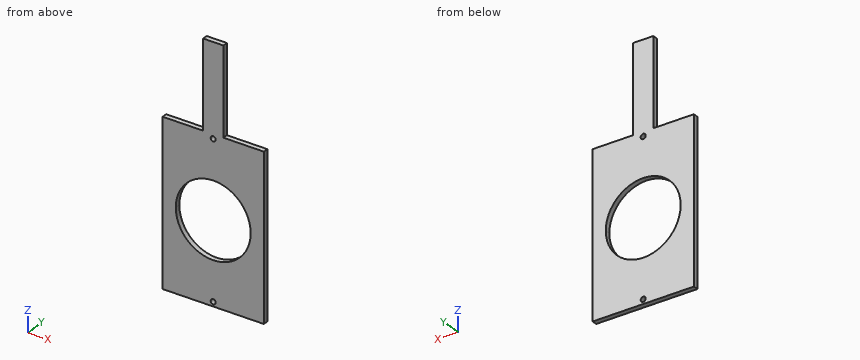
from build123d import *

# Parameters (mm, degrees)
F1_DEPTH = 3.175


# Not quite as in the source:
# - a feature names something its author has since deleted; it is built from what else it names


with BuildPart() as f1:
    # F0 (on Front) → F1 (new body)
    with BuildSketch(Plane.XZ):
        with BuildLine():
            Line((-94.8762850642, 108.0007998444), (-120.2762850642, 108.0007998444))
            Line((-120.2762850642, 108.0007998444), (-120.2762850642, 57.2007998444))
            Line((-120.2762850642, 57.2007998444), (-112.0251095462, 57.2007998444))
            ThreePointArc((-112.0251095462, 57.2007998444), (-105.1424632053, 73.8169779855), (-88.5262850642, 80.6996243264))
            Line((-88.5262850642, 80.6996243264), (-88.5262850642, 103.6132998444))
            ThreePointArc((-88.5262850642, 103.6132998444), (-90.1137850642, 105.2007998444), (-88.5262850642, 106.7882998444))
            Line((-88.5262850642, 106.7882998444), (-88.5262850642, 108.0007998444))
            Line((-88.5262850642, 108.0007998444), (-94.8762850642, 108.0007998444))
        make_face()
        with BuildLine():
            Line((-82.1762850642, 108.0007998444), (-88.5262850642, 108.0007998444))
            Line((-88.5262850642, 108.0007998444), (-88.5262850642, 106.7882998444))
            ThreePointArc((-88.5262850642, 106.7882998444), (-87.4037530491, 106.3233318595), (-86.9387850642, 105.2007998444))
            ThreePointArc((-86.9387850642, 105.2007998444), (-87.4037530491, 104.0782678293), (-88.5262850642, 103.6132998444))
            Line((-88.5262850642, 103.6132998444), (-88.5262850642, 80.6996243264))
            ThreePointArc((-88.5262850642, 80.6996243264), (-71.9101069231, 73.8169779855), (-65.0274605822, 57.2007998444))
            ThreePointArc((-65.0274605822, 57.2007998444), (-71.9101069231, 40.5846217033), (-88.5262850642, 33.7019753624))
            Line((-88.5262850642, 33.7019753624), (-88.5262850642, 10.7882998444))
            ThreePointArc((-88.5262850642, 10.7882998444), (-87.4037530491, 10.3233318595), (-86.9387850642, 9.2007998444))
            ThreePointArc((-86.9387850642, 9.2007998444), (-87.4037530491, 8.0782678293), (-88.5262850642, 7.6132998444))
            Line((-88.5262850642, 7.6132998444), (-88.5262850642, 6.4007998444))
            Line((-88.5262850642, 6.4007998444), (-56.7762850642, 6.4007998444))
            Line((-56.7762850642, 6.4007998444), (-56.7762850642, 108.0007998444))
            Line((-56.7762850642, 108.0007998444), (-82.1762850642, 108.0007998444))
        make_face()
        with BuildLine():
            Line((-112.0251095462, 57.2007998444), (-120.2762850642, 57.2007998444))
            Line((-120.2762850642, 57.2007998444), (-120.2762850642, 6.4007998444))
            Line((-120.2762850642, 6.4007998444), (-88.5262850642, 6.4007998444))
            Line((-88.5262850642, 6.4007998444), (-88.5262850642, 7.6132998444))
            ThreePointArc((-88.5262850642, 7.6132998444), (-90.1137850642, 9.2007998444), (-88.5262850642, 10.7882998444))
            Line((-88.5262850642, 10.7882998444), (-88.5262850642, 33.7019753624))
            ThreePointArc((-88.5262850642, 33.7019753624), (-105.1424632053, 40.5846217033), (-112.0251095462, 57.2007998444))
        make_face()
        Polygon((-94.8762850642, 162.3507998444), (-94.8762850642, 108.0007998444), (-88.5262850642, 108.0007998444), (-82.1762850642, 108.0007998444), (-82.1762850642, 162.3507998444), align=None)
    extrude(amount=F1_DEPTH)


solid = f1.part
The listing builds one solid part. Answer for the finished solid, in the listing's coordinates (mm). Give positions to 0.01 mm unless a question says otherwise; leave off trailing zeros. Order: outer loops, then holes, each group sorted by start corner. A loop starts at its lowest first (then second) coordinate and runs counter-clockwise, first axis right, second up. Notation, with made-up numbers: (56.5, -37.5) - (70.5, -37.5) arc R34 cw to (70.5, 0.5) - close; hole circle Ø8 at (-5, 69.5). An arc over 180 degrees is marked (long way). Use one line per item in the form item = value.
1) Find section A-A on z = 70. Determine the outline of the cut face in (x, y) (3 decimals), and give its area (3 significant figures).
Verdict:
outline = (-120.276, -3.175) - (-108.234, -3.175) - (-108.234, 0) - (-120.276, 0) - close; (-68.819, -3.175) - (-56.776, -3.175) - (-56.776, 0) - (-68.819, 0) - close
area = 76.5 mm^2
2) Consider probe 1 along Z at (x, y) = (-89, -1.05); probe 2 along X at (y, z) = (-2, 130.5); probe 3 along Z at (x, y) = (-108, -1.05). Determine where each line is inside the solid, lowest interval first. Write a range as [from, to].
Verdict:
probe_1 = [6.4, 7.69], [10.72, 33.71], [80.69, 103.69], [106.72, 162.35]
probe_2 = [-94.88, -82.18]
probe_3 = [6.4, 44.05], [70.35, 108]
3) Find section B-B on y = -2.65. Determine the outline of the cut face in (x, z) (1 decimal).
Verdict:
outline = (-120.3, 6.4) - (-56.8, 6.4) - (-56.8, 108) - (-82.2, 108) - (-82.2, 162.4) - (-94.9, 162.4) - (-94.9, 108) - (-120.3, 108) - close; hole circle Ø47 at (-88.5, 57.2); hole circle Ø3.2 at (-88.5, 9.2); hole circle Ø3.2 at (-88.5, 105.2)
4) Find section C-C on x = -104.5. Determine the outline of the cut face in (y, z) (1 decimal), and give its area (3 significant figures).
Verdict:
outline = (-3.2, 6.4) - (0, 6.4) - (0, 40) - (-3.2, 40) - close; (-3.2, 74.4) - (0, 74.4) - (0, 108) - (-3.2, 108) - close
area = 213 mm^2
5) This flat-tipped pin is pushed along its axis until it touches: pin 1 (1 mm diameter, centred on y = -2, z = 135, fed in from +X). Where does it stop, or does it pass through?
Verdict:
pin_1 = -82.18
6) Find section D-D on z = 131. Determine the outline of the cut face in (x, y) (3 decimals), and give its area (3 significant figures).
Verdict:
outline = (-94.876, -3.175) - (-82.176, -3.175) - (-82.176, 0) - (-94.876, 0) - close
area = 40.3 mm^2
